Design review of the part built by this model. Coordinates are the model's own, in mm. Coordinates: 2 decimals unless noted, no trailing zeros. Write each loop counter-clockwise with the first axis right and the second up, starting at its lowest first coordinate (ties: lowest second). Pieces come first, ordered by that corner, then holes. Notation, with made-up numbers: (1.5, 41.25) -> (52.5, 41.25) arc R24 cw to (52.5, 72.25) -> close; hole circle Ø7 at (73.25, -10.75). An arc over 180 degrees is marked (long way). One line per question, with ' | ' between items. Start each with the question number.
Q1. Wall thickness on probe 1 along Y at (x, z) = (-5.5, 1.35); probe 2 along X at (y, z) = (-16.5, 0.25); probe 3 along Y at (x, z) = (-15.5, 2.65): over which ranges is each line inside the solid? List them lowest first.
Q2. Add section C-C on x = -7.5. State the section outline as (y, z) points.
Q3. Add section A-A on x = 0. State the section outline as (y, z) points.
Q4. Add section D-D on z = 1.75. State the section outline as (x, y) points.
Q5. Add section B-B on y = 34. State the section outline as (x, z) points.
from build123d import *

# Parameters (mm, degrees)
SKETCH_W      = 60.084118
SKETCH_H      = 80.392258
SKETCH_R      = 9.312632
SKETCH_R_2    = 7.062198
SKETCH_W_2    = 20.62126
SKETCH_H_2    = 10.683233
EXTRUDE_DEPTH = 4


with BuildPart() as part:
    # Sketch → Extrude (new body)
    with BuildSketch(Plane.XY):
        Rectangle(SKETCH_W, SKETCH_H)
        with Locations((-15.149905, 25.553061)):
            Circle(SKETCH_R, mode=Mode.SUBTRACT)
        with Locations((15.781789, 22.447472)):
            Circle(SKETCH_R_2, mode=Mode.SUBTRACT)
        with Locations((0, -15.092993)):
            Rectangle(SKETCH_W_2, SKETCH_H_2, mode=Mode.SUBTRACT)
    extrude(amount=EXTRUDE_DEPTH)


solid = part.part
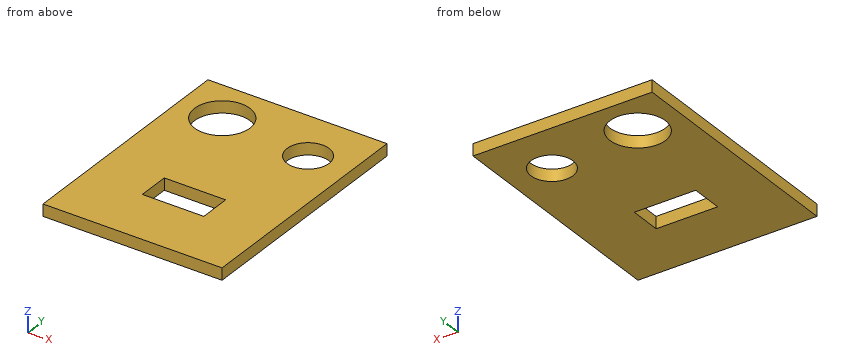
Output values:
1) probe 1: y = -40.2 to -20.43, -9.75 to 40.2 | probe 2: x = -30.04 to -10.31, 10.31 to 30.04 | probe 3: y = -40.2 to 16.25, 34.86 to 40.2
2) outline: (-40.2, 0) -> (-20.43, 0) -> (-20.43, 4) -> (-40.2, 4) -> close; (-9.75, 0) -> (20.24, 0) -> (20.24, 4) -> (-9.75, 4) -> close; (30.86, 0) -> (40.2, 0) -> (40.2, 4) -> (30.86, 4) -> close
3) outline: (-40.2, 0) -> (-20.43, 0) -> (-20.43, 4) -> (-40.2, 4) -> close; (-9.75, 0) -> (40.2, 0) -> (40.2, 4) -> (-9.75, 4) -> close
4) outline: (-30.04, -40.2) -> (30.04, -40.2) -> (30.04, 40.2) -> (-30.04, 40.2) -> close; hole circle Ø18.63 at (-15.15, 25.55); hole (-10.31, -20.43) -> (10.31, -20.43) -> (10.31, -9.75) -> (-10.31, -9.75) -> close; hole circle Ø14.12 at (15.78, 22.45)
5) outline: (-30.04, 0) -> (-19.07, 0) -> (-19.07, 4) -> (-30.04, 4) -> close; (-11.23, 0) -> (30.04, 0) -> (30.04, 4) -> (-11.23, 4) -> close
